Part print with two shaded views. Sizes in mm from the minimum x, y, z corner. A direction names the side the tool comes from. Give positions to 0.01 mm unless a question says otherwise; leave off trailing zeros. Loops run counter-clockwise (first coordinate to the right, second up) from the corner with the lowest first, then second, coordinate; pieces in that order, holes last. Notation, with made-up numbers: M 87.5,2.5 L 130.5,2.5 A27 cw 130.5,31.5 Z; hole C 3,43 d7. An arc over 180 degrees is marked long. Answer as a JSON object with one key per item and string values. Group by question number.
1. Mould opens along Y. For the marked faces 4, 5, 6 and 7 say: released by +Y, released by -Y, zero draft, split by the parting line, or undercut.
2. Slice it at B-B (z = 31.5). List the corners of the cut face in (x, y) (1 decimal).
3. Slice it at A-A (x = 2.5). List the corners of the cut face in (y, z) (1 decimal).
4. Slice it at D-D (y = 23). List the corners of the cut face in (x, z).
5. Drop flat-ended pins along their axis: pin 1 Ø12 at (y, z) = (32.5, 75) entering from -X; pin 2 Ø6 at (x, y) = (7, 19) entering from -Z. Give the stop position or say it passes through.
6. Drill centre lines: line 1 along Y through (x, z) = (19, 46.5) (1 decimal); line 2 along Y through (x, z) = (4, 15.5) (1 decimal); line 3 along Z through (x, y) = (23.5, 15.5). Where is each one in solid material? Low to high. Write a range as [from, to].
7. Slice it at C-C (y = 54.5). List the corners of the cut face in (x, z).
8. 3-axis set-ups, long thin cutter, end or side, ignore diameter. For the marked faces 1, 2 and 3: which of +Z, -Z, +X, -X, +Y, -Y reach the whole face in a straight line?
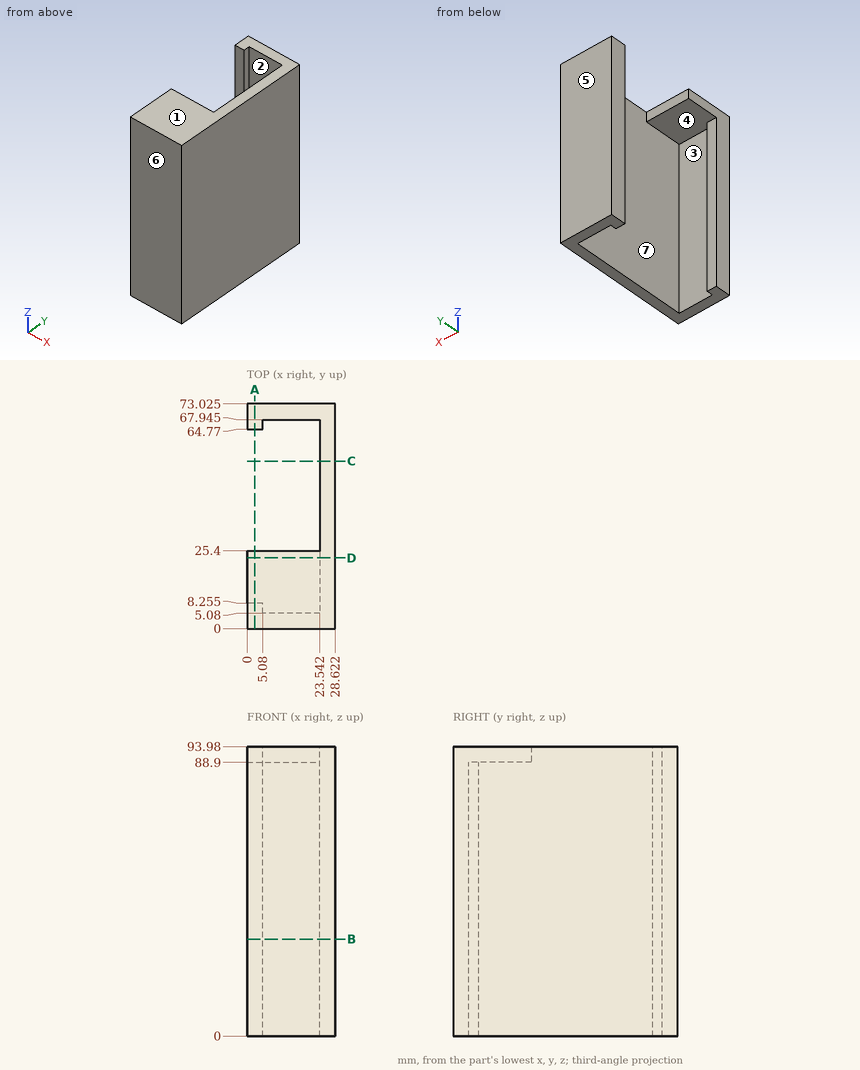
Established:
{
 "1": {"face 4": "undercut", "face 5": "released by +Y", "face 6": "released by -Y", "face 7": "undercut"},
 "2": {"outline": "M 0,0 L 28.6,0 L 28.6,73 L 0,73 L 0,64.8 L 5.1,64.8 L 5.1,67.9 L 23.5,67.9 L 23.5,5.1 L 5.1,5.1 L 5.1,8.3 L 0,8.3 Z"},
 "3": {"outline": "M 0,0 L 8.3,0 L 8.3,88.9 L 25.4,88.9 L 25.4,94 L 0,94 Z; M 64.8,0 L 73,0 L 73,94 L 64.8,94 Z"},
 "4": {"outline": "M 0,88.9 L 23.54,88.9 L 23.54,0 L 28.62,0 L 28.62,93.98 L 0,93.98 Z"},
 "5": {"pin 1": "stops at x = 23.54", "pin 2": "stops at z = 88.9"},
 "6": {"line 1": "y = [0, 5.1], [67.9, 73]", "line 2": "y = [0, 8.3], [64.8, 73]", "line 3": "z = [88.9, 93.98]"},
 "7": {"outline": "M 23.54,0 L 28.62,0 L 28.62,93.98 L 23.54,93.98 Z"},
 "8": {"face 1": "+Z, +X, -X, +Y, -Y", "face 2": "+Z, -Z", "face 3": "-Z"}
}
